Input: part model. Units: mm. Frame: model coordinates. Round coordinates to 2 decimals unless told otherwise and drop trailing zeros. Write each loop counter-clockwise with the first axis right and the second up, starting at its lowest first coordinate (ties: lowest second). Pieces come first, ordered by that corner, then holes. Notation, with made-up numbers: (19.5, 81) -> (78.5, 81) arc R28 cw to (78.5, 104) -> close; hole circle Ø8 at (66, -23.75). An arc over 180 degrees is marked (long way). Use CSV: the item, a comma, the result in double quotes.
```python
from build123d import *

# Parameters (mm, degrees)
SKETCH1_W           = 23
SKETCH1_H           = 6
SKETCH2_R           = 26
SKETCH2_R_2         = 1
BOSS_EXTRUDE1_DEPTH = 0.5
BOSS_EXTRUDE2_START = 0.5
SKETCH3_R           = 26
BOSS_EXTRUDE2_DEPTH = 0.5
SKETCH4_R           = 1
CUT_EXTRUDE2_DEPTH  = 7
SKETCH5_R           = 4
CUT_EXTRUDE3_DEPTH  = 10


with BuildPart() as part:
    # Sketch1 → Revolve1 (revolve)
    with BuildSketch(Plane(origin=(0, 0, 0), x_dir=(1, 0, 0), z_dir=(0, 1, 0))):
        with BuildLine():
            Line((23, 6), (23, 3))
            ThreePointArc((23, 3), (23.878679656, 5.121320344), (26, 6))
            Line((26, 6), (23, 6))
        make_face()
        with BuildLine():
            Line((23, 3), (23, 0))
            Line((23, 0), (26, 0))
            ThreePointArc((26, 0), (23.878679656, 0.878679656), (23, 3))
        make_face()
        with Locations((11.5, 3)):
            Rectangle(SKETCH1_W, SKETCH1_H)
    revolve(axis=Axis((0, 0, 0), (0, 0, -1)))

    # Sketch2 → Boss-Extrude1 (add)
    with BuildSketch(Plane.XY):
        Circle(SKETCH2_R)
        Circle(SKETCH2_R_2, mode=Mode.SUBTRACT)
    extrude(amount=BOSS_EXTRUDE1_DEPTH)

    # Sketch3 → Boss-Extrude2 (add)
    with BuildSketch(Plane(origin=(0, 0, -6), x_dir=(-1, 0, 0), z_dir=(0, 0, -1)).offset(BOSS_EXTRUDE2_START)):
        with Locations(Location((0, 0, 0), (0, 0, 180))):
            Circle(SKETCH3_R)
    extrude(amount=-BOSS_EXTRUDE2_DEPTH)

    # Sketch4 → Cut-Extrude2 (cut)
    with BuildSketch(Plane(origin=(0, 0, -6.5), x_dir=(-1, 0, 0), z_dir=(0, 0, -1))):
        Circle(SKETCH4_R)
    extrude(amount=-CUT_EXTRUDE2_DEPTH, mode=Mode.SUBTRACT)

    # Sketch5 → Cut-Extrude3 (cut)
    with BuildSketch(Plane(origin=(0, 0, -6.5), x_dir=(-1, 0, 0), z_dir=(0, 0, -1))):
        Circle(SKETCH5_R)
    extrude(amount=-CUT_EXTRUDE3_DEPTH, mode=Mode.SUBTRACT)


solid = part.part
```
Item 1: Section query A-A on z = -2.25. Return the cut outline in (x, y).
Worked answers:
outline,"circle Ø46.19 at (0, 0); hole circle Ø8 at (0, 0)"
Item 2: First-contact query: pin 1 Ø2 at (x, z) = (-12, -2) entering from +Y; pin 2 Ø1 at (y, z) = (1, -2.5) entering from -X; pin 3 Ø1 at (x, z) = (-4, -3) entering from -Y. Flat tips, straight axial feed; report the tip coordinate or a pass-through.
Worked answers:
pin 1,"stops at y = 20.67"
pin 2,"stops at x = -23.15"
pin 3,"stops at y = -22.73"
Item 3: Section query B-B on z = -5.25. Return the cut outline in (x, y).
Worked answers:
outline,"circle Ø48.03 at (0, 0); hole circle Ø8 at (0, 0)"
Item 4: Pull-direction query (X, two-part tool) for faces 1 (the face through (0.867, -3.905, -3.049)), 2 (the face through (5, 0, -6.5)), 3 (the face through (-20.633, -15.821, 0.246)); classes: +X half, -X half, draft (parallel to the pull), parting line (faces both ways), or undercut.
Worked answers:
face 1,"undercut"
face 2,"draft"
face 3,"parting line"
Item 5: Line query: line 1 (Z direction, x = 2, y = 24); line 2 (Y direction, x = 0, z = -4.5); line 3 (Z direction, x = 7.5, y = 23.5). Output: solid intervals per line, ascending.
Worked answers:
line 1,"z = -6.5 to -5.31, -0.69 to 0.5"
line 2,"y = -23.4 to -4, 4 to 23.4"
line 3,"z = -6.5 to -5.69, -0.31 to 0.5"
